The listing builds one solid part. Answer for the finished solid, in the listing's coordinates (mm). A direction names the side the tool comes from. Round coordinates to 2 decimals unless told otherwise and drop trailing zeros. Write each loop counter-clockwise with the first axis right and the second up, starting at its lowest first coordinate (ties: lowest second). Pieces come first, ordered by that corner, then holes.
Item 1: Find section C-C on y = -94.5. Give the vertices of the cut face in (x, z).
Item 2: For a pull along X with two mould halves and no side action, classify faces 1 (the face through (48, 0, 6)), 2 (the face through (48, -25.367, 31)), 3 (the face through (-52.473, -50, 31)) as +X half, -X half, draft (parallel to the pull), parting line (faces both ways), or undercut.
Item 3: Find the intervals of material crossed by probe 1 along X at (y, z) = (-39.5, 28.5); probe 2 along Y at (x, z) = (-5.5, 34.5); probe 3 along Z at (x, y) = (69.5, -76.5), in increasing order.
Item 4: A tool of negligible diameter and unlimited length cuts with its end or side. For faces 4 (the face through (-27.073, -64, 31)), 5 (the face through (-52.592, -50, -14)), from which of +Z, -Z, +X, -X, +Y, -Y can it reach the whole face along a straight path? Write none if from no direction.
Item 5: Find section B-B on x = 56.5. Give the vertices of the cut face in (y, z).
Item 6: Find section A-A on z = 39.5. Give the vertices of the cut face in (x, y).
Item 7: Each of these flat-tipped pins is pushed along its axis until it touches: pin 1 (4 mm diameter, centred on x = 49, z = -22.5, fed in from -Y); pin 2 (19.5 mm diameter, centred on x = 42, z = 37, fed in from -Y); pin 3 (12 mm diameter, centred on y = -53.5, z = -25, fed in from +X). Where does it stop, or does it pass through?
```python
from build123d import *

# Parameters (mm, degrees)
F0_W     = 203.2
F0_H     = 50.8
F1_DEPTH = 101.6
F2_W     = 25.4
F2_H     = 25.3674704581
F2_W_2   = 152.3310508887
F2_H_2   = 76.2325295419
F2_W_3   = 0.2561658621
F2_W_4   = 25.2127832492
F2_H_3   = 0.0325295419
F3_DEPTH = 50.8


with BuildPart() as f1:
    # F0 (on Front) → F1 (new body)
    with BuildSketch(Plane.XZ):
        with Locations((49.0080691226, -13.7808406726)):
            Rectangle(F0_W, F0_H)
    extrude(amount=F1_DEPTH)

    # F2 (on Top) → F3 (join)
    with BuildSketch(Plane.XY):
        with Locations((-39.7728137652, -12.6837352291)):
            Rectangle(F2_W, F2_H)
        with Locations((49.0927116791, -12.6837352291)):
            Rectangle(F2_W_2, F2_H)
        with Locations((-39.7728137652, -63.4837352291)):
            Rectangle(F2_W, F2_H_2)
        with Locations((125.3863200545, -12.6837352291)):
            Rectangle(F2_W_3, F2_H)
        Polygon((125.5144029856, -25.3674704581), (125.2582371235, -25.3674704581), (125.2582371235, -102.1268442273), (150.7271862348, -102.1268442273), (150.7271862348, -25.4), (125.5144029856, -25.4), align=None)
        with Locations((138.1207946102, -12.6837352291)):
            Rectangle(F2_W_4, F2_H)
        with Locations((138.1207946102, -25.3837352291)):
            Rectangle(F2_W_4, F2_H_3)
    extrude(amount=F3_DEPTH)


solid = f1.part
```
Check values:
1. outline: (-52.59, -39.18) - (150.61, -39.18) - (150.61, 0) - (150.73, 0) - (150.73, 50.8) - (125.26, 50.8) - (125.26, 11.62) - (-27.07, 11.62) - (-27.07, 50.8) - (-52.47, 50.8) - (-52.47, 11.62) - (-52.59, 11.62) - close
2. face 1: draft
2. face 2: undercut
2. face 3: -X half
3. probe 1: x = -52.47 to -27.07, 125.26 to 150.73
3. probe 2: y = -25.37 to 0
3. probe 3: z = -39.18 to 11.62
4. face 4: +Z, -Y
4. face 5: +Z, -Z, -X, +Y, -Y
5. outline: (-101.6, -39.18) - (0, -39.18) - (0, 50.8) - (-25.37, 50.8) - (-25.37, 11.62) - (-101.6, 11.62) - close
6. outline: (-52.47, -101.6) - (-27.07, -101.6) - (-27.07, -25.37) - (125.26, -25.37) - (125.26, -102.13) - (150.73, -102.13) - (150.73, 0) - (-52.47, 0) - close
7. pin 1: stops at y = -101.6
7. pin 2: stops at y = -25.37
7. pin 3: stops at x = 150.61
